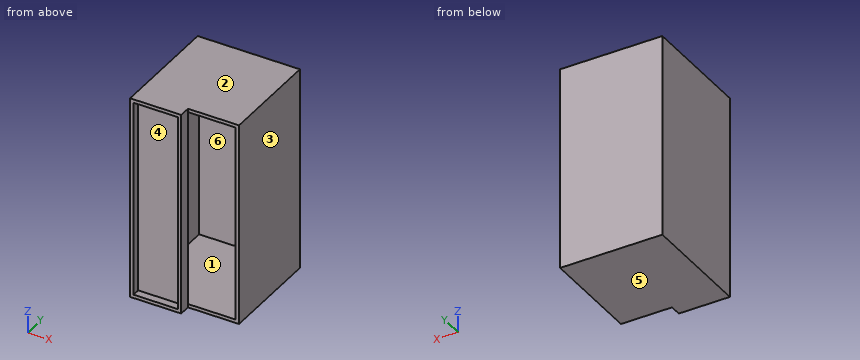
from build123d import *

# Parameters (mm, degrees)
F0_W         = 75.8234336972
F0_H         = 151.4142677188
F1_DEPTH     = 75.946
F3_T         = -2.54
F2_W         = 37.9117168486
F2_H         = 151.4142677188
F4_DEPTH     = 8.382
F5_T         = 2.54
F5_T3_DEPTH  = 7.62
F5_T5_DEPTH  = 7.62
F5_T7_DEPTH  = 40.4517168486
F5_T9_DEPTH  = 151.4142677188
F5_T11_DEPTH = 78.486
F5_T13_DEPTH = 75.8234336972


# Not quite as in the source:
# - a shell that OpenCascade refuses in one call is made with other operations: the cavity is built on its own and cut out


with BuildPart() as f1:
    # F0 (on Front) → F1 (new body)
    with BuildSketch(Plane.XZ):
        with Locations((-37.9117168486, -0.1162923872)):
            Rectangle(F0_W, F0_H)
    extrude(amount=F1_DEPTH)

    # F3
    f3_openings = [f1.faces().sort_by_distance(p)[0] for p in [
        (-37.911717, -75.946, -0.116292),
    ]]
    offset(amount=F3_T, openings=f3_openings)

    # F2 (on face) → F4 (join)
    with BuildSketch(Plane.XZ.offset(75.946)):
        with Locations((-56.8675752729, -0.1162923872)):
            Rectangle(F2_W, F2_H)
    extrude(amount=F4_DEPTH)

    # F5: shell of thickness 2.54, made by hand


with BuildPart() as f5_core1:
    # F5_t2: copy of F1
    add(f1.part)

    # the walls: a layer under each face that stays
    f5_faces = [f5_core1.faces().sort_by_distance(p)[0] for p in [
        (-37.9117168486, -42.164, 75.5908414721),
        (-37.9117168486, 0, -0.1162923872),
        (-37.9117168486, -42.164, -75.8234262466),
        (-75.8234336972, -42.164, -0.1162923872),
        (-37.9117168486, -80.137, -0.1162923872),
        (-55.5975752729, -75.946, -0.1162923872),
        (-37.9117168486, -39.243, 73.0508414721),
        (-2.54, -39.243, -0.1162923872),
        (-37.9117168486, -2.54, -0.1162923872),
        (-73.2834336972, -39.243, -0.1162923872),
        (-37.9117168486, -39.243, -73.2834262466),
        (-1.263723895, -75.946, -70.7762839894),
        (0, -37.973, -0.1162923872),
    ]]
    thicken(f5_faces, amount=-F5_T, mode=Mode.SUBTRACT)

    # F5_s4 → F5_t3 (cut)
    with BuildSketch(Plane.XY.offset(-78.3634262466)):
        Polygon((-37.8863168486, -75.9714), (-40.4517168486, -75.946), (-40.4517168486, -73.406), (-37.9117168486, -73.406), align=None)
    extrude(amount=F5_T3_DEPTH, mode=Mode.SUBTRACT)

    # F5_s6 → F5_t5 (cut)
    with BuildSketch(Plane.XY.offset(70.5108414721)):
        Polygon((-37.8863168486, -75.9714), (-40.4517168486, -75.946), (-40.4517168486, -73.406), (-37.9117168486, -73.406), align=None)
    extrude(amount=F5_T5_DEPTH, mode=Mode.SUBTRACT)

    # F5_s8 → F5_t7 (cut)
    with BuildSketch(Plane.YZ.offset(-75.8234336972)):
        Polygon((-75.9206, -73.2580262466), (-78.486, -73.2834262466), (-78.486, -75.8234262466), (-75.946, -75.8234262466), align=None)
        Polygon((-75.9206, 73.0254414721), (-78.486, 73.0508414721), (-78.486, 75.5908414721), (-75.946, 75.5908414721), align=None)
    extrude(amount=F5_T7_DEPTH, mode=Mode.SUBTRACT)

    # F5_s10 → F5_t9 (cut)
    with BuildSketch(Plane.XY.offset(-75.8234262466)):
        Polygon((-73.2580336972, -75.9206), (-73.2834336972, -78.486), (-75.8234336972, -78.486), (-75.8234336972, -75.946), align=None)
        Polygon((-2.5654, -2.5654), (0, -2.54), (0, 0), (-2.54, 0), align=None)
        Polygon((-73.2580336972, -2.5654), (-73.2834336972, 0), (-75.8234336972, 0), (-75.8234336972, -2.54), align=None)
    extrude(amount=F5_T9_DEPTH, mode=Mode.SUBTRACT)

    # F5_s12 → F5_t11 (cut)
    with BuildSketch(Plane.XZ):
        Polygon((-73.2580336972, 73.0254414721), (-73.2834336972, 75.5908414721), (-75.8234336972, 75.5908414721), (-75.8234336972, 73.0508414721), align=None)
        Polygon((-2.5654, 73.0254414721), (-2.54, 75.5908414721), (0, 75.5908414721), (0, 73.0508414721), align=None)
        Polygon((-2.5654, -73.2580262466), (0, -73.2834262466), (0, -75.8234262466), (-2.54, -75.8234262466), align=None)
        Polygon((-73.2580336972, -73.2580262466), (-75.8234336972, -73.2834262466), (-75.8234336972, -75.8234262466), (-73.2834336972, -75.8234262466), align=None)
    extrude(amount=F5_T11_DEPTH, mode=Mode.SUBTRACT)

    # F5_s14 → F5_t13 (cut)
    with BuildSketch(Plane.YZ.offset(-75.8234336972)):
        Polygon((-2.5654, 73.0254414721), (-2.54, 75.5908414721), (0, 75.5908414721), (0, 73.0508414721), align=None)
        Polygon((-2.5654, -73.2580262466), (0, -73.2834262466), (0, -75.8234262466), (-2.54, -75.8234262466), align=None)
    extrude(amount=F5_T13_DEPTH, mode=Mode.SUBTRACT)


with BuildPart() as f1_1:
    add(f1.part)

    # what is left inside the walls is the cavity
    f5_cavity = [f5_core1.part.solids().sort_by_distance(p)[0] for p in [
        (-56.867575, -78.5114, -24.505337),
    ]]
    add(f5_cavity, mode=Mode.SUBTRACT)


solid = f1_1.part
Read the model definition and answer for the solid it produces. Units are mm, in the model's axes. Face numbers are marked on the shaded views. A direction names the side the tool comes from. Round coordinates to 2 decimals unless told otherwise and drop trailing zeros. Write each loop counter-clockwise with the first axis right and the second up, starting at its lowest first coordinate (ties: lowest second). Pieces come first, ordered by that corner, then holes. Notation, with made-up numbers: (27, 88) - (72, 88) arc R20 cw to (72, 101) - close; hole circle Ø7 at (-7.75, -5). An arc over 180 degrees is marked (long way). Use a Markdown table: item, result.
(1) Straight lines are drawn through the part: line 1 along X through (y, z) = (-28.5, 22); line 2 along Y through (x, z) = (-52, 54); line 3 along Z through (x, y) = (-61.5, -41.5). For each, find the intervals that lie inside material, in ascending order. Write a range as [from, to].
Reported:
| item | result |
|---|---|
| line 1 | [-75.82, -73.28], [-2.54, 0] |
| line 2 | [-78.49, -75.95], [-2.54, 0] |
| line 3 | [-75.82, -73.28], [73.05, 75.59] |
(2) The part is cut by section C-C (z = -9.5). Write down the section's boundary in (x, y), then the cut area to 3 significant figures.
Reported:
| item | result |
|---|---|
| outline | (-75.82, -84.33) - (-73.28, -84.33) - (-73.28, -78.49) - (-40.45, -78.49) - (-40.45, -84.33) - (-37.91, -84.33) - (-37.91, -75.95) - (-73.28, -75.95) - (-73.28, -2.54) - (-2.54, -2.54) - (-2.54, -75.95) - (0, -75.95) - (0, 0) - (-75.82, 0) - close |
| area | 691 mm2 |
(3) Each of these flat-tipped pins is pushed along its axis until it touches: pin 1 Ø1.8 at (y, z) = (-81, 8.5) entering from +X; pin 2 Ø6 at (x, z) = (-47.5, -58) entering from -Y; pin 3 Ø19 at (x, z) = (-13, -24.5) entering from -Y. Where does it stop, or does it pass through?
Reported:
| item | result |
|---|---|
| pin 1 | x = -37.91 |
| pin 2 | y = -78.49 |
| pin 3 | y = -2.54 |
(4) The part is cut by section B-B (y = -41). Write down the section's boundary in (x, z).
Reported:
| item | result |
|---|---|
| outline | (-75.82, -75.82) - (0, -75.82) - (0, 75.59) - (-75.82, 75.59) - close; hole (-73.28, -73.28) - (-2.54, -73.28) - (-2.54, 73.05) - (-73.28, 73.05) - close |
(5) The part is cut by section A-A (x = -68). Write down the section's boundary in (y, z).
Reported:
| item | result |
|---|---|
| outline | (-84.33, -75.82) - (0, -75.82) - (0, 75.59) - (-84.33, 75.59) - (-84.33, 73.05) - (-78.49, 73.05) - (-78.49, -73.28) - (-84.33, -73.28) - close; hole (-75.95, -73.28) - (-2.54, -73.28) - (-2.54, 73.05) - (-75.95, 73.05) - close |
(6) The mould has two halves that part along X. Classify the marked faces 3, 4, 5 and 6: released by +X, released by -X, zero draft, split by the parting line, or undercut.
Reported:
| item | result |
|---|---|
| face 3 | released by +X |
| face 4 | undercut |
| face 5 | zero draft |
| face 6 | undercut |
(7) Which of the six approach directions +Z, -Z, +X, -X, +Y, -Y give full straight-line access (tool end or side, diameter ignored) to the marked faces 1 and 2?
Reported:
| item | result |
|---|---|
| face 1 | none |
| face 2 | +Z, +X, -X, +Y, -Y |
(8) The part is cut by section D-D (x = -18.5). Write down the section's boundary in (y, z).
Reported:
| item | result |
|---|---|
| outline | (-75.95, -75.82) - (0, -75.82) - (0, 75.59) - (-75.95, 75.59) - (-75.95, 73.05) - (-2.54, 73.05) - (-2.54, -73.28) - (-75.95, -73.28) - close |
